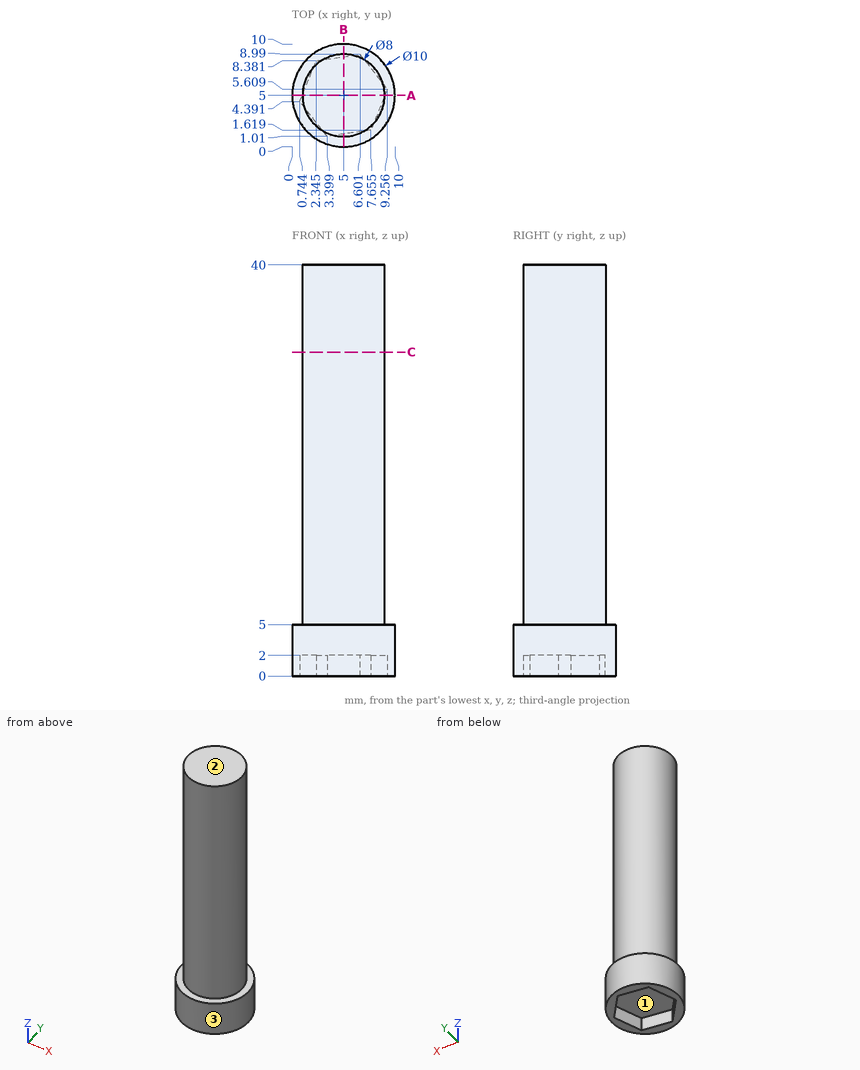
Source: three-view drawing plus pictorial views. Frame: mm from the lowest corner of the part. Give positions to 0.01 mm unless a question says otherwise; leave off trailing zeros. Write each loop counter-clockwise with the first axis right and the second up, starting at its lowest first coordinate (ties: lowest second). Pieces come first, ordered by that corner, then holes. Notation, with made-up numbers: (10, 44) -> (34, 44) arc R22 ccw to (34, 56) -> close; hole circle Ø1 at (-23, -3). An arc over 180 degrees is marked (long way). Answer in a Markdown table with one row per item.
(1) Draft query along Y for the marked faces 1, 2 and 3. Return one class per face: +Y half, -Y half, draft (parallel to the pull), parting line (faces both ways), or undercut.
Answers below:
| item | result |
|---|---|
| face 1 | undercut |
| face 2 | draft |
| face 3 | parting line |
(2) Section query A-A on y = 5. Return loops of the section in (x, z).
Answers below:
| item | result |
|---|---|
| outline | (0, 0) -> (0.99, 0) -> (0.99, 2) -> (9.01, 2) -> (9.01, 0) -> (10, 0) -> (10, 5) -> (9, 5) -> (9, 40) -> (1, 40) -> (1, 5) -> (0, 5) -> close |
(3) Ray query, line 1 along Z through (x, y) = (3, 1.25); line 2 along Y through (x, z) = (5, 9); line 3 along Z through (x, y) = (5, 6). Return the intervals inside material, ascending. Write a range as [from, to].
Answers below:
| item | result |
|---|---|
| line 1 | [0, 5] |
| line 2 | [1, 9] |
| line 3 | [2, 40] |
(4) Pin query (flat end, axial travel): pin 1 (2.5 mm diameter, centred on x = 4, y = 6.5, fed in from -Z); pin 2 (5 mm diameter, centred on y = 3.5, z = 9, fed in from +X); pin 3 (3 mm diameter, centred on y = 7.5, z = 32, fed in from -X). Return the tip coordinate at first contact, or that it passes through.
Answers below:
| item | result |
|---|---|
| pin 1 | z = 2 |
| pin 2 | x = 9 |
| pin 3 | x = 1.13 |
(5) Section query B-B on x = 5. Return loops of the section in (y, z), then the cut area to 3 significant figures.
Answers below:
| item | result |
|---|---|
| outline | (0, 0) -> (1.24, 0) -> (1.24, 2) -> (8.76, 2) -> (8.76, 0) -> (10, 0) -> (10, 5) -> (9, 5) -> (9, 40) -> (1, 40) -> (1, 5) -> (0, 5) -> close |
| area | 315 mm^2 |
(6) Section query C-C on z = 31.5. Return loops of the section in (x, y).
Answers below:
| item | result |
|---|---|
| outline | circle Ø8 at (5, 5) |
